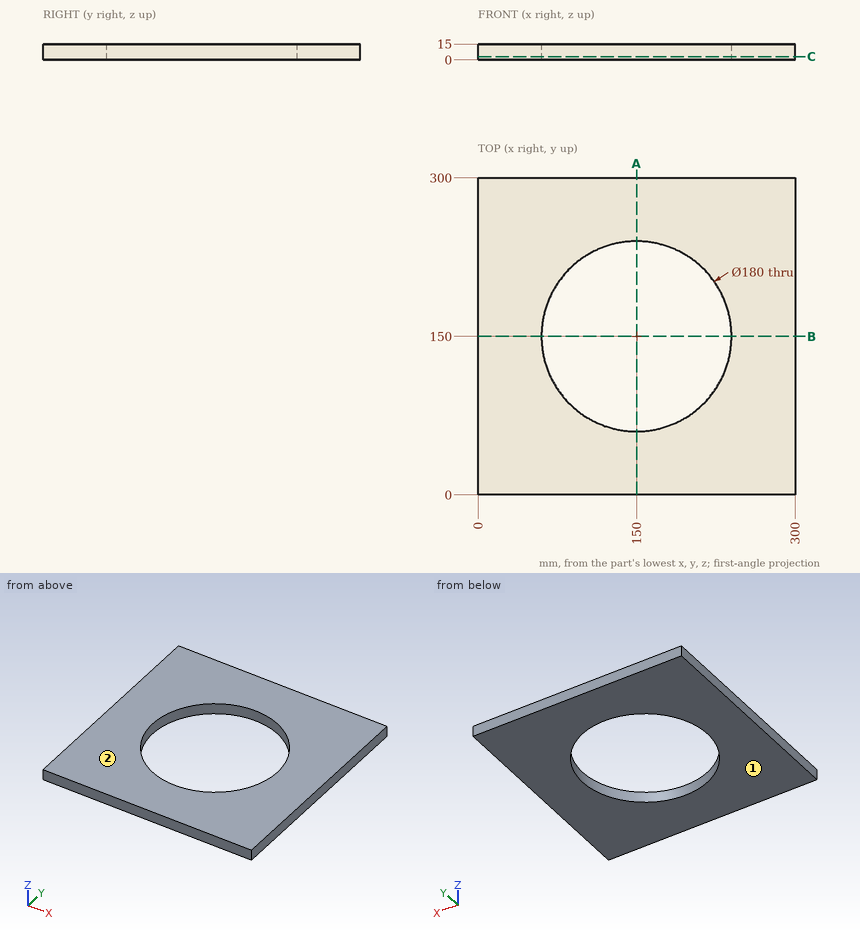
Geometry check sheet. Reference: drawing and pictorial views, mm from the part's lowest x, y, z. Give positions to 0.01 mm unless a question says otherwise; leave off trailing zeros. Write each loop counter-clockwise with the first axis right and the second up, starting at its lowest first coordinate (ties: lowest second). Pieces come first, ordered by that corner, then holes. Notation, with made-up numbers: (67.5, -25) - (126.5, -25) arc R21 cw to (126.5, -12) - close; hole circle Ø9 at (-37, -12.75). An arc over 180 degrees is marked (long way). Use a Markdown table: item, result.
Q1. Section check A-A, the plane x = 150. Enter the section's corners in (y, z), then the cut area to 3 significant figures.
Computed:
| item | result |
|---|---|
| outline | (0, 0) - (60, 0) - (60, 15) - (0, 15) - close; (240, 0) - (300, 0) - (300, 15) - (240, 15) - close |
| area | 1,800 mm² |
Q2. Section check C-C, the plane z = 3. Enter the section's corners in (x, y).
Computed:
| item | result |
|---|---|
| outline | (0, 0) - (300, 0) - (300, 300) - (0, 300) - close; hole circle Ø180 at (150, 150) |
Q3. Thickness scan on L1, parallel to Y at x = 150, z = 9.5; L2, parallel to Y at x = 120.5, z = 5.5; L3, parallel to X at y = 84.5, z = 5. Record the ranges inside material, lowest first. Write a range as [from, to].
Computed:
| item | result |
|---|---|
| L1 | y = [0, 60], [240, 300] |
| L2 | y = [0, 64.97], [235.03, 300] |
| L3 | x = [0, 88.28], [211.72, 300] |
Q4. Draft check along Z on the marked faces 1 and 2. Enter one of: pulls with the +Z half, pulls with the -Z half, needs draft (parallel to the pull), parting line crosses it, or undercut.
Computed:
| item | result |
|---|---|
| face 1 | pulls with the -Z half |
| face 2 | pulls with the +Z half |
